Part print with two shaded views. Sizes in mm from the minimum x, y, z corner. A direction names the side the tool comes from. Give positions to 0.01 mm unless a question says otherwise; leave off trailing zeros. Write each loop counter-clockwise with the first axis right and the second up, starting at its lowest first coordinate (ties: lowest second). Pieces come first, ordered by that corner, then holes.
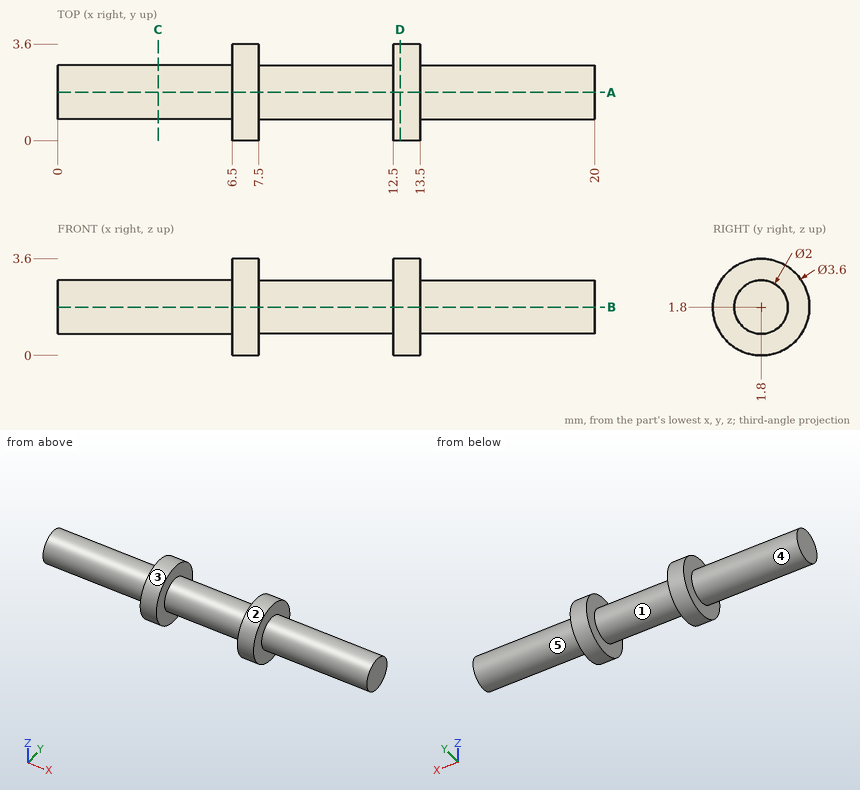
1) 3-axis set-ups, long thin cutter, end or side, ignore diameter. For the marked faces 3, 4 and 5: which of +Z, -Z, +X, -X, +Y, -Y reach the whole face in a straight line?
Answers follow:
face 3: +X, -X
face 4: -X
face 5: +X
2) Saw through at D-D, the plane x = 12.75. Write the cut outline in (y, z).
Answers follow:
outline: circle Ø3.6 at (1.8, 1.8)
3) Saw through at A-A, the plane y = 1.8. Write the cut outline in (x, z), then the cut area to 3 significant figures.
Answers follow:
outline: (0, 0.8) - (6.5, 0.8) - (6.5, 0) - (7.5, 0) - (7.5, 0.8) - (12.5, 0.8) - (12.5, 0) - (13.5, 0) - (13.5, 0.8) - (20, 0.8) - (20, 2.8) - (13.5, 2.8) - (13.5, 3.6) - (12.5, 3.6) - (12.5, 2.8) - (7.5, 2.8) - (7.5, 3.6) - (6.5, 3.6) - (6.5, 2.8) - (0, 2.8) - close
area: 43.2 mm2
4) Two-plate mould, pull along X, no slides. Class the marked faces 1 and 2: +X half, -X half, draft (parallel to the pull), parting line (faces both ways), or undercut.
Answers follow:
face 1: undercut
face 2: draft
5) Saw through at C-C, the plane x = 3.75. Write the cut outline in (y, z).
Answers follow:
outline: circle Ø2 at (1.8, 1.8)
6) Wall check: L1, parallel to X at y = 0.65, z = 0.5; L2, parallel to Z at x = 3.25, y = 1.9; L3, parallel to Y at x = 14.25, z = 1.85. Give the ranges that are in metal, low to high.
Answers follow:
L1: x = 6.5 to 7.5, 12.5 to 13.5
L2: z = 0.81 to 2.79
L3: y = 0.8 to 2.8
7) Pin check, flat tips, straight feed: pin 1 Ø2 at (x, z) = (2.5, 0.5) entering from +Y; pin 2 Ø1.5 at (x, y) = (17.5, 2) entering from +Z. Stop position of each tip, or through.
Answers follow:
pin 1: stops at y = 2.75
pin 2: stops at z = 2.8
